from build123d import *

# Parameters (mm, degrees)
BOSS_EXTRUDE2_DEPTH   = 40
BOSS_EXTRUDE2_2_DEPTH = 40
BOSS_EXTRUDE2_3_DEPTH = 40
BOSS_EXTRUDE2_4_DEPTH = 40
BOSS_EXTRUDE2_5_DEPTH = 40
BOSS_EXTRUDE3_DEPTH   = 40
SKETCH3_R             = 7.5
BOSS_EXTRUDE4_DEPTH   = 40
SKETCH5_R             = 5.5
BOSS_EXTRUDE5_DEPTH   = 5
SKETCH4_R             = 3.45
CUT_EXTRUDE1_DEPTH    = 45


with BuildPart() as part:
    # Sketch1 → Boss-Extrude2 (new body)
    with BuildSketch(Plane(origin=(0, 0, 0), x_dir=(1, 0, 0), z_dir=(0, 1, 0))):
        with BuildLine():
            Line((0, 17.5), (0, 15))
            ThreePointArc((0, 15), (6.339273926, 13.594616806), (11.490666647, 9.641814145))
            Line((11.490666647, 9.641814145), (13.405777755, 11.24878317))
            ThreePointArc((13.405777755, 11.24878317), (7.39581958, 15.860386273), (0, 17.5))
        make_face()
    extrude(amount=BOSS_EXTRUDE2_DEPTH)



with BuildPart() as body_2:
    # Sketch1 → Boss-Extrude2 2 (new body)
    with BuildSketch(Plane(origin=(0, 0, 0), x_dir=(1, 0, 0), z_dir=(0, 1, 0))):
        with BuildLine():
            Line((16.643489035, 5.407797402), (14.265847744, 4.635254916))
            ThreePointArc((14.265847744, 4.635254916), (14.888192275, -1.828040151), (12.720721442, -7.948788963))
            Line((12.720721442, -7.948788963), (14.840841683, -9.273587124))
            ThreePointArc((14.840841683, -9.273587124), (17.369557654, -2.13271351), (16.643489035, 5.407797402))
        make_face()
    extrude(amount=BOSS_EXTRUDE2_2_DEPTH)


with BuildPart() as body_3:
    # Sketch1 → Boss-Extrude2 3 (new body)
    with BuildSketch(Plane(origin=(0, 0, 0), x_dir=(1, 0, 0), z_dir=(0, 1, 0))):
        with BuildLine():
            Line((10.286241915, -14.157797402), (8.816778784, -12.135254916))
            ThreePointArc((8.816778784, -12.135254916), (2.862134931, -14.724407752), (-3.628828434, -14.554435894))
            Line((-3.628828434, -14.554435894), (-4.233633173, -16.98017521))
            ThreePointArc((-4.233633173, -16.98017521), (3.339157419, -17.17847571), (10.286241915, -14.157797402))
        make_face()
    extrude(amount=BOSS_EXTRUDE2_3_DEPTH)


with BuildPart() as body_4:
    # Sketch1 → Boss-Extrude2 4 (new body)
    with BuildSketch(Plane(origin=(0, 0, 0), x_dir=(1, 0, 0), z_dir=(0, 1, 0))):
        with BuildLine():
            Line((-10.286241915, -14.157797402), (-8.816778784, -12.135254916))
            ThreePointArc((-8.816778784, -12.135254916), (-13.119295607, -7.272144304), (-14.963460754, -1.046347106))
            Line((-14.963460754, -1.046347106), (-17.45737088, -1.220738291))
            ThreePointArc((-17.45737088, -1.220738291), (-15.305844875, -8.484168354), (-10.286241915, -14.157797402))
        make_face()
    extrude(amount=BOSS_EXTRUDE2_4_DEPTH)


with BuildPart() as body_5:
    # Sketch1 → Boss-Extrude2 5 (new body)
    with BuildSketch(Plane(origin=(0, 0, 0), x_dir=(1, 0, 0), z_dir=(0, 1, 0))):
        with BuildLine():
            Line((-16.643489035, 5.407797402), (-14.265847744, 4.635254916))
            ThreePointArc((-14.265847744, 4.635254916), (-10.970305524, 10.229975401), (-5.619098901, 13.907757819))
            Line((-5.619098901, 13.907757819), (-6.555615385, 16.225717455))
            ThreePointArc((-6.555615385, 16.225717455), (-12.798689778, 11.934971301), (-16.643489035, 5.407797402))
        make_face()
    extrude(amount=BOSS_EXTRUDE2_5_DEPTH)


with BuildPart() as part_1:
    add(part.part)

    add(body_2.part)  # Boss-Extrude3 merges body 2

    add(body_3.part)  # Boss-Extrude3 merges body 3

    add(body_4.part)  # Boss-Extrude3 merges body 4

    add(body_5.part)  # Boss-Extrude3 merges body 5
    # Sketch2 → Boss-Extrude3 (add)
    with BuildSketch(Plane(origin=(0, 0, 0), x_dir=(1, 0, 0), z_dir=(0, 1, 0))):
        Polygon((-1.438002264, -3.083805807), (0.898880564, -15.106025742), (4.825389298, -14.342789761), (2.48850647, -2.320569825), (14.644453588, -3.813132454), (15.131930961, 0.157052152), (2.975983844, 1.649614781), (8.1518895, 12.749380282), (4.526658352, 14.439853329), (-0.649247305, 3.340087828), (-9.606308804, 11.692682804), (-12.334302244, 8.767267998), (-3.377240745, 0.414673022), (-14.088914848, -5.522904889), (-12.149676367, -9.021383718), align=None)
        Polygon((-0.334260109, 0.311702594), (0.152686649, 0.084635592), (0.087207921, -0.448645859), align=None, mode=Mode.SUBTRACT)
    extrude(amount=BOSS_EXTRUDE3_DEPTH)

    # Sketch3 → Boss-Extrude4 (add)
    with BuildSketch(Plane(origin=(0, 0, 0), x_dir=(1, 0, 0), z_dir=(0, 1, 0))):
        Circle(SKETCH3_R)
    extrude(amount=BOSS_EXTRUDE4_DEPTH)

    # Sketch5 → Boss-Extrude5 (add)
    with BuildSketch(Plane(origin=(0, 40, 0), x_dir=(1, 0, 0), z_dir=(0, 1, 0))):
        Circle(SKETCH5_R)
    extrude(amount=BOSS_EXTRUDE5_DEPTH)

    # Sketch4 → Cut-Extrude1 (cut)
    with BuildSketch(Plane(origin=(0, 0, 0), x_dir=(1, 0, 0), z_dir=(0, 1, 0))):
        Circle(SKETCH4_R)
    extrude(amount=CUT_EXTRUDE1_DEPTH, mode=Mode.SUBTRACT)


solid = part_1.part
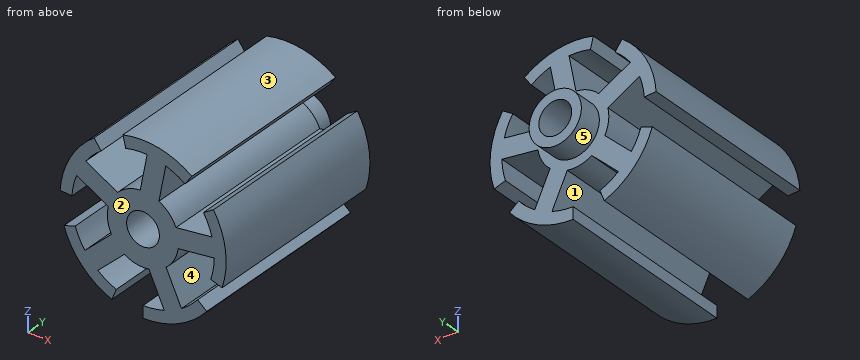
Verification items for the finished model (mm, model axes). Face numbers are marked on the shaded views. A direction names the side the tool comes from. Round coordinates to 2 decimals unless told otherwise and drop trailing zeros. Use a Markdown table: item, result. Add a question column.
1. Gauge pin test, flat ends, axial feed: pin 1 (10 mm diameter, centred on x = -9.5, z = 9, fed in from +Y); pin 2 (4 mm diameter, centred on x = -5.5, y = 12.5, fed in from +Z); pin 3 (1.5 mm diameter, centred on x = -10.5, y = 38.5, fed in from +Z). Record the tip position at first contact, or that the pin passes through.
2. Access from +Z, -Z, +X, -X, +Y, -Y to the whole of each face (thin tool, end or side, straight path). Record for the marked faces 1 and 2.
3. Release check for a two-part mould opening along Z. For the marked faces 3, 4 and 5 record: released by +Z, released by -Z, zero draft, split by the parting line, or undercut.
4. Thickness scan on probe 1 along X at (y, z) = (20.5, 0); probe 2 along X at (y, z) = (36, -10.5); probe 3 along Z at (x, y) = (9, 10). Record the ranges inside material, lowest first. Write a range as [from, to].
Checks:
| question | item | result |
|---|---|---|
| 1 | pin 1 | stops at y = 40 |
| 1 | pin 2 | stops at z = 17.15 |
| 1 | pin 3 | stops at z = 14.16 |
| 2 | face 1 | +Y, -Y |
| 2 | face 2 | +Z, -Z, +X, -X, -Y |
| 3 | face 3 | released by +Z |
| 3 | face 4 | undercut |
| 3 | face 5 | split by the parting line |
| 4 | probe 1 | x = [-7.5, -3.45], [3.45, 17.5] |
| 4 | probe 2 | x = [-14, -8.33], [2.69, 7.1], [10.71, 12.51] |
| 4 | probe 3 | z = [-15.01, -12], [-0.91, 3.12], [12.39, 15.01] |
